Read the model definition and answer for the solid it produces. Units are mm, in the model's axes. A direction names the side the tool comes from. Round coordinates to 2 decimals unless told otherwise and drop trailing zeros. Write each loop counter-clockwise with the first axis right and the second up, starting at its lowest first coordinate (ties: lowest second). Pieces come first, ordered by that corner, then holes.
from build123d import *

# Parameters (mm, degrees)
SKETCH2_R           = 39.487475
BOSS_EXTRUDE1_DEPTH = 5.842
FILLET1_R           = 0.79375
CUT_EXTRUDE2_DEPTH  = 163.986308211
CIRPATTERN2_COUNT   = 3


with BuildPart() as part:
    # Sketch2 → Boss-Extrude1 (new body)
    with BuildSketch(Plane(origin=(0, 0, 0), x_dir=(0, 0, -1), z_dir=(1, 0, 0))):
        with BuildLine():
            Line((81.02619141, 88.258519733), (35.921024484, 114.3))
            ThreePointArc((35.921024484, 114.3), (0, 63.5), (-35.921024484, 114.3))
            Line((-35.921024484, 114.3), (-81.02619141, 88.258519733))
            ThreePointArc((-81.02619141, 88.258519733), (-54.99261314, 31.75), (-116.947215895, 26.041480267))
            Line((-116.947215895, 26.041480267), (-116.947215895, -26.041480267))
            ThreePointArc((-116.947215895, -26.041480267), (-54.99261314, -31.75), (-81.02619141, -88.258519733))
            Line((-81.02619141, -88.258519733), (-35.921024484, -114.3))
            ThreePointArc((-35.921024484, -114.3), (0, -63.5), (35.921024484, -114.3))
            Line((35.921024484, -114.3), (81.02619141, -88.258519733))
            ThreePointArc((81.02619141, -88.258519733), (54.99261314, -31.75), (116.947215895, -26.041480267))
            Line((116.947215895, -26.041480267), (116.947215895, 26.041480267))
            ThreePointArc((116.947215895, 26.041480267), (54.99261314, 31.75), (81.02619141, 88.258519733))
        make_face()
        Circle(SKETCH2_R, mode=Mode.SUBTRACT)
    extrude(amount=BOSS_EXTRUDE1_DEPTH)

    # Fillet1
    fillet1_edges = [part.edges().sort_by_distance(p)[0] for p in [
        (2.921, 88.258519733, 81.02619141),
        (2.921, 114.3, 35.921024484),
        (2.921, 114.3, -35.921024484),
        (2.921, 88.258519733, -81.02619141),
        (2.921, 26.041480267, -116.947215895),
        (2.921, -26.041480267, -116.947215895),
        (2.921, -88.258519733, -81.02619141),
        (2.921, -114.3, -35.921024484),
        (2.921, -114.3, 35.921024484),
        (2.921, -88.258519733, 81.02619141),
        (2.921, -26.041480267, 116.947215895),
        (2.921, 26.041480267, 116.947215895),
    ]]
    fillet(fillet1_edges, radius=FILLET1_R)

    # Sketch6 → Cut-Extrude2 (cut, through all)
    with BuildSketch(Plane(origin=(5.842, 0, 0), x_dir=(0, 0, -1), z_dir=(1, 0, 0))):
        with BuildLine():
            Line((-23.004455913, 45.686886441), (-29.096698147, 56.238959523))
            ThreePointArc((-29.096698147, 56.238959523), (-29.144557493, 56.602487346), (-29.367768813, 56.311592689))
            Line((-29.367768813, 56.311592689), (-34.08338539, 53.589030189))
            ThreePointArc((-34.08338539, 53.589030189), (-34.446913212, 53.541170844), (-34.156018556, 53.317959523))
            Line((-34.156018556, 53.317959523), (-28.004456056, 42.663140727))
            ThreePointArc((-28.004456056, 42.663140727), (-27.954648068, 42.299101356), (-27.735435356, 42.593976392))
            Line((-27.735435356, 42.593976392), (-23.075039112, 45.412346944))
            ThreePointArc((-23.075039112, 45.412346944), (-22.713049707, 45.465623764), (-23.004455913, 45.686886441))
        make_face()
    cut_extrude2 = extrude(amount=-CUT_EXTRUDE2_DEPTH, mode=Mode.SUBTRACT)

    # CirPattern2: Cut-Extrude2 ×3 about axis
    cirpattern2_axis = Axis((0, 0, 0), (1, 0, 0))
    for i in range(1, CIRPATTERN2_COUNT):
        add(cut_extrude2.rotate(cirpattern2_axis, i * 360 / CIRPATTERN2_COUNT), mode=Mode.SUBTRACT)


solid = part.part
Q1. Flat-ended cylindrical pins translate along their axes: pin 1 Ø1 at (x, z) = (2, -61) entering from +Y; pin 2 Ø8 at (y, z) = (-27, 65) entering from +X; pin 3 Ø5 at (y, z) = (-56.5, -41.5) entering from -X; pin 4 Ø1 at (x, z) = (1.5, -28) entering from +Y. Find the tip coordinate at first contact, or state that the pin passes through.
Verdict:
pin 1: stops at y = 100.11
pin 2: passes through
pin 3: stops at x = 0
pin 4: stops at y = 76.31
Q2. Straight lines are drawn through the part: probe 1 along Y at (x, z) = (1.2, -71.5); probe 2 along Y at (x, z) = (1.45, -59.5); probe 3 along Z at (x, y) = (5.05, -103.5). For each, find the intervals that lie inside material, in ascending order.
Verdict:
probe 1: y = -93.76 to -85.15, -16.45 to 16.45, 85.15 to 93.76
probe 2: y = -100.69 to -76.1, -25.5 to -2.92, 2.92 to 25.5, 76.1 to 100.69
probe 3: z = -54.63 to -38.05, 38.05 to 54.63
Q3. Which of the six approach directions +Z, -Z, +X, -X, +Y, -Y give full straight-line access (tool end or side, diameter ignored) to faces 1 (the flat face through (2.96, 50.89, 26.01)), 2 (the flat face through (5.842, 34, 27))?
Verdict:
face 1: +X, -X
face 2: +Z, -Z, +X, +Y, -Y
Q4. Section C-C (z = 56.5) is taken. Determine the outline of the cut face in (x, y).
Verdict:
outline: (0, -102.42) - (5.84, -102.42) - (5.84, -72.25) - (0, -72.25) - close; (0, -29.35) - (5.84, -29.35) - (5.84, 29.35) - (0, 29.35) - close; (0, 72.25) - (5.84, 72.25) - (5.84, 102.42) - (0, 102.42) - close
Q5. Determine the mould class of faces 3 (the flat face through (2.88, 101.45, 58.18)), 4 (the flat face through (3, 0, 116.947)), 5 (the cylindrical face through (2.9, 30.9, -55.5)) for opening direction Y: pulls with the +Y half, pulls with the -Y half, needs draft (parallel to the pull), parting line crosses it, or undercut.
Verdict:
face 3: pulls with the +Y half
face 4: needs draft
face 5: undercut
Q6. Section D-D (y = 101.6) is taken. Determine the outline of the cut face in (x, z).
Verdict:
outline: (0, -57.92) - (5.84, -57.92) - (5.84, -38.1) - (0, -38.1) - close; (0, 38.1) - (5.84, 38.1) - (5.84, 57.92) - (0, 57.92) - close
Q7. Section B-B (y = 0) is taken. Determine the outline of the cut face in (x, z).
Verdict:
outline: (0, -116.95) - (5.84, -116.95) - (5.84, -63.45) - (0, -63.45) - close; (0, -50.81) - (5.84, -50.81) - (5.84, -39.49) - (0, -39.49) - close; (0, 39.49) - (5.84, 39.49) - (5.84, 116.95) - (0, 116.95) - close
Q8. Section A-A (z = 0) is taken. Determine the outline of the cut face in (x, y).
Verdict:
outline: (0, -63.5) - (5.84, -63.5) - (5.84, -39.49) - (0, -39.49) - close; (0, 39.49) - (5.84, 39.49) - (5.84, 63.5) - (0, 63.5) - close
